from build123d import *

# Parameters (mm, degrees)
SKETCH1_R           = 2.05
BOSS_EXTRUDE1_DEPTH = 2.25
CUT_EXTRUDE2_DEPTH  = 3


with BuildPart() as part:
    # Sketch1 → Boss-Extrude1 (new, symmetric)
    with BuildSketch(Plane.XY):
        with BuildLine():
            Line((-20, -18), (20, -18))
            ThreePointArc((20, -18), (22.828427125, -16.828427125), (24, -14))
            Line((24, -14), (24, 14))
            ThreePointArc((24, 14), (22.828427125, 16.828427125), (20, 18))
            Line((20, 18), (-20, 18))
            ThreePointArc((-20, 18), (-22.828427125, 16.828427125), (-24, 14))
            Line((-24, 14), (-24, -14))
            ThreePointArc((-24, -14), (-22.828427125, -16.828427125), (-20, -18))
        make_face()
        with Locations((-20, -14)):
            Circle(SKETCH1_R, mode=Mode.SUBTRACT)
        with Locations((-20, 14)):
            Circle(SKETCH1_R, mode=Mode.SUBTRACT)
        with Locations((20, 14)):
            Circle(SKETCH1_R, mode=Mode.SUBTRACT)
        with Locations((20, -14)):
            Circle(SKETCH1_R, mode=Mode.SUBTRACT)
    extrude(amount=BOSS_EXTRUDE1_DEPTH, both=True)

    # Sketch3 → Cut-Extrude2 (cut)
    with BuildSketch(Plane.XY.offset(2.25)):
        with BuildLine():
            Line((23, -14), (23, 14))
            ThreePointArc((23, 14), (22.121320344, 16.121320344), (20, 17))
            Line((20, 17), (-20, 17))
            ThreePointArc((-20, 17), (-22.121320344, 16.121320344), (-23, 14))
            Line((-23, 14), (-23, -14))
            ThreePointArc((-23, -14), (-22.121320344, -16.121320344), (-20, -17))
            Line((-20, -17), (20, -17))
            ThreePointArc((20, -17), (22.121320344, -16.121320344), (23, -14))
        make_face()
    extrude(amount=-CUT_EXTRUDE2_DEPTH, mode=Mode.SUBTRACT)


solid = part.part
Can you work these out from the model? Positions are in its coordinate system, mm. A direction names the side the tool comes from. Give positions to 0.01 mm unless a question says otherwise; leave off trailing zeros. Loops run counter-clockwise (first coordinate to the right, second up) from the corner with the lowest first, then second, coordinate; pieces in that order, holes last. Notation, with made-up numbers: (34, -15) -> (57, -15) arc R14 ccw to (57, -2) -> close; hole circle Ø5 at (-36.75, 30.5). An arc over 180 degrees is marked (long way). Use one line per item in the form item = value.
1) We'd pull the mould along X, two halves only. Please class faces 3 (the face through (22.797, -16.859, 0.031)), 4 (the face through (-20.444, 11.999, -1.51)), 5 (the face through (-24, 0, 0)), 6 (the face through (0, 0, -2.25)): released by +X, released by -X, zero draft, split by the parting line, or undercut.
Answers:
face_3 = released by +X
face_4 = undercut
face_5 = released by -X
face_6 = zero draft
2) If we section it at A-A (z = 1.5): Please give me the cut outline in (x, y), plus the area to 3 significant figures.
Answers:
outline = (-24, -14) arc R4 ccw to (-20, -18) -> (20, -18) arc R4 ccw to (24, -14) -> (24, 14) arc R4 ccw to (20, 18) -> (-20, 18) arc R4 ccw to (-24, 14) -> close; hole (-23, -14) arc R3 ccw to (-20, -17) -> (20, -17) arc R3 ccw to (23, -14) -> (23, 14) arc R3 ccw to (20, 17) -> (-20, 17) arc R3 ccw to (-23, 14) -> close
area = 158 mm²
3) I need wall thicknesses on line 1 along X through (y, z) = (14, -1.2); line 2 along Y through (x, z) = (20, -1.35); line 3 along X through (y, z) = (6.5, 1.05). Which ranges of each line are inside material? Lowest first, please.
Answers:
line_1 = -24 to -22.05, -17.95 to 17.95, 22.05 to 24
line_2 = -18 to -16.05, -11.95 to 11.95, 16.05 to 18
line_3 = -24 to -23, 23 to 24
4) Will these pins go through, and if not, where does the flat tip stop? pin 1 (5.5 mm diameter, centred on x = -20, y = 14, fed in from -Z); pin 2 (1 mm diameter, centred on x = -14.5, y = -10, fed in from +Z); pin 3 (3.5 mm diameter, centred on x = 20, y = -14, fed in from +Z).
Answers:
pin_1 = -2.25
pin_2 = -0.75
pin_3 = through
5) If we section it at B-B (x = -10): Please give me the cut outline in (y, z).
Answers:
outline = (-18, -2.25) -> (18, -2.25) -> (18, 2.25) -> (17, 2.25) -> (17, -0.75) -> (-17, -0.75) -> (-17, 2.25) -> (-18, 2.25) -> close
6) For faces 1 (the face through (-23, 0, 1)), 2 (the face through (-23.2, 0.1, 2.25)), which set-ups out of +Z, -Z, +X, -X, +Y, -Y let a thin tool reach every point of the face, with its end or its side?
Answers:
face_1 = +Z
face_2 = +Z, +X, -X, +Y, -Y
7) If we section it at C-C (y = -4.5): Please give me the cut outline in (x, z).
Answers:
outline = (-24, -2.25) -> (24, -2.25) -> (24, 2.25) -> (23, 2.25) -> (23, -0.75) -> (-23, -0.75) -> (-23, 2.25) -> (-24, 2.25) -> close
